```python
from build123d import *

# Parameters (mm, degrees)
BOSS_EXTRUDE1_DEPTH = 11.5
SKETCH2_W           = 16.8
SKETCH2_H           = 15.6
BOSS_EXTRUDE2_DEPTH = 2
BOSS_EXTRUDE3_DEPTH = 2


with BuildPart() as part:
    # Sketch1 → Boss-Extrude1 (new body)
    with BuildSketch(Plane(origin=(0, 0, 0), x_dir=(1, 0, 0), z_dir=(0, 1, 0))):
        Polygon((-8.4, 8.4), (-8.4, -7.2), (-7.2, -7.2), (-7.2, 7.2), (7.2, 7.2), (7.2, -7.2), (8.4, -7.2), (8.4, 8.4), align=None)
    extrude(amount=BOSS_EXTRUDE1_DEPTH)

    # Sketch2 → Boss-Extrude2 (add)
    with BuildSketch(Plane.XZ):
        with Locations((0, -0.6)):
            Rectangle(SKETCH2_W, SKETCH2_H)
    extrude(amount=BOSS_EXTRUDE2_DEPTH)

    # Sketch3 → Boss-Extrude3 (add)
    with BuildSketch(Plane(origin=(0, 11.5, 0), x_dir=(1, 0, 0), z_dir=(0, 1, 0))):
        with BuildLine():
            Line((-4, 0), (-4, -7.2))
            Line((-4, -7.2), (-8.4, -7.2))
            Line((-8.4, -7.2), (-8.4, 8.4))
            Line((-8.4, 8.4), (8.4, 8.4))
            Line((8.4, 8.4), (8.4, -7.2))
            Line((8.4, -7.2), (4, -7.2))
            Line((4, -7.2), (4, 0))
            ThreePointArc((4, 0), (0, 4), (-4, 0))
        make_face()
    extrude(amount=BOSS_EXTRUDE3_DEPTH)


solid = part.part
```
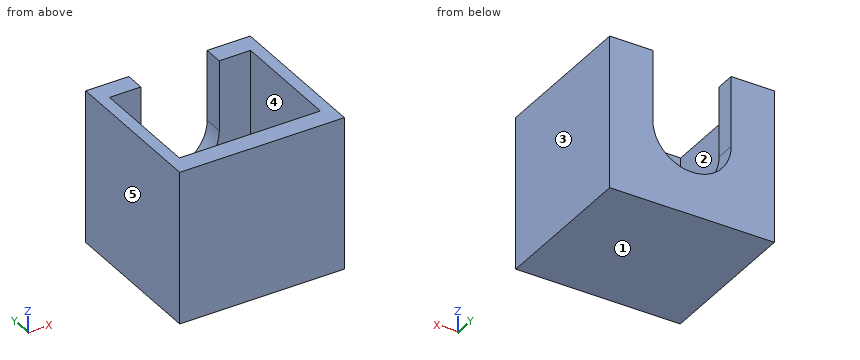
Geometry check sheet. Reference: the model listing, model coordinates, mm. Face numbers are marked on the shaded views. A direction names the side the tool comes from. Round coordinates to 2 decimals unless told otherwise and drop trailing zeros. Order: outer loops, then holes, each group sorted by start corner. A loop starts at its lowest first (then second) coordinate and runs counter-clockwise, first axis right, second up. Notation, with made-up numbers: (64.25, 85) - (114.25, 85) arc R9 cw to (114.25, 99) - close; hole circle Ø9 at (74, 15). An arc over 180 degrees is marked (long way). Use a Markdown table: item, result. Add a question column.
(1) Sectioned sample at A-A, the plane z = -4.5. Enter the section's corners in (x, y).
(2) Tool access check on the marked faces 4 and 5. Record the directions out of +Z, -Z, +X, -X, +Y, -Y that give a thin tool (end or side, any length) a straight path to the whole face; none if there is none.
(3) Sectioned sample at B-B, the plane y = 1. Enter the section's corners in (x, z).
(4) Release check for a two-part mould opening along X. For the marked faces 1, 2 and 3 record: pulls with the +X half, pulls with the -X half, needs draft (parallel to the pull), parting line crosses it, or undercut.
(5) Material ranges on line 1 along X through (y, z) = (5.5, 4); line 2 along Y through (x, z) = (-5.75, -6.5); line 3 along Z through (x, y) = (5.75, 5.5), recorded low to high. Write a range as [from, to].
(6) Sectioned sample at D-D, the plane z = -1. Enter the section's corners in (x, y).
(7) Sectioned sample at C-C, the plane x = 6.75. Enter the section's corners in (y, z).
Answers below:
| question | item | result |
|---|---|---|
| 1 | outline | (-8.4, -2) - (8.4, -2) - (8.4, 13.5) - (-8.4, 13.5) - close; hole (-7.2, 0) - (7.2, 0) - (7.2, 11.5) - (-7.2, 11.5) - close |
| 2 | face 4 | +Z |
| 2 | face 5 | +Z, -Z, -X, +Y, -Y |
| 3 | outline | (-8.4, -8.4) - (8.4, -8.4) - (8.4, 7.2) - (7.2, 7.2) - (7.2, -7.2) - (-7.2, -7.2) - (-7.2, 7.2) - (-8.4, 7.2) - close |
| 4 | face 1 | needs draft |
| 4 | face 2 | undercut |
| 4 | face 3 | pulls with the +X half |
| 5 | line 1 | [-8.4, -7.2], [7.2, 8.4] |
| 5 | line 2 | [-2, 0], [11.5, 13.5] |
| 5 | line 3 | [-8.4, -7.2] |
| 6 | outline | (-8.4, -2) - (8.4, -2) - (8.4, 13.5) - (3.87, 13.5) - (3.87, 11.5) - (7.2, 11.5) - (7.2, 0) - (-7.2, 0) - (-7.2, 11.5) - (-3.87, 11.5) - (-3.87, 13.5) - (-8.4, 13.5) - close |
| 7 | outline | (-2, -8.4) - (13.5, -8.4) - (13.5, 7.2) - (11.5, 7.2) - (11.5, -7.2) - (0, -7.2) - (0, 7.2) - (-2, 7.2) - close |
